Geometry check sheet. Reference: the model listing, model coordinates, mm. A direction names the side the tool comes from. Round coordinates to 2 decimals unless told otherwise and drop trailing zeros. Order: outer loops, then holes, each group sorted by start corner. A loop starts at its lowest first (then second) coordinate and runs counter-clockwise, first axis right, second up. Notation, with made-up numbers: (65, 79.25) - (105, 79.25) arc R10 ccw to (105, 86.25) - close; hole circle Ø2 at (-32.5, 67). An arc over 180 degrees is marked (long way). Return JSON: item names as keys, results as strings. Group by question number.
Q1. Draft check along Y on faces 6 (the flat face through (113.5, 13, 5)), 7 (the flat face through (-2, 2, -10)), 8 (the flat face through (-2, 0, 0)), 9 (the flat face through (-2, 26, 5)). Enter one of: pulls with the +Y half, pulls with the -Y half, needs draft (parallel to the pull), parting line crosses it, or undercut.
Q2. Sectioned sample at B-B, the plane x = 70. Record the cut outline in (y, z), then the cut area to 3 significant figures.
Q3. Sectioned sample at A-A, the plane y = 15.75. Record the cut outline in (x, z), then the cut area to 3 significant figures.
Q4. Material ranges on line 1 along X through (y, z) = (9.25, 1); line 2 along Z through (x, y) = (-26.9, 2.35); line 3 along Y through (x, z) = (-119.5, 3.5), recorded low to high.
Q5. Gauge pin test, flat ends, axial feed: pin 1 Ø6.5 at (x, y) = (-58.5, 20.5) entering from -Z; pin 2 Ø1 at (x, z) = (-17, -1.5) entering from +Y. Record the tip position at first contact, or that the pin passes through.
Q6. Tool access check on faces 1 (the flat face through (-2, 16, 0)), 2 (the flat face through (-2, 5, -4)), 3 (the flat face through (-2, 13, 10)), 4 (the flat face through (134.5, 13, 5)), 5 (the flat face through (121, 21, 5)). Record the directions out of +Z, -Z, +X, -X, +Y, -Y that give a thin tool (end or side, any length) a straight path to the whole face; none if there is none.
```python
from build123d import *

# Parameters (mm, degrees)
SKETCH_W     = 269
SKETCH_H     = 26
SKETCH_W_2   = 16
SKETCH_H_2   = 16
PAD_DEPTH    = 10
SKETCH002_W  = 269
SKETCH002_H  = 5
PAD001_DEPTH = 10
SKETCH003_R  = 1.5
POCKET_DEPTH = 5.001


with BuildPart() as part:
    # Sketch → Pad (new body)
    with BuildSketch(Plane.XY):
        with Locations((0, 13)):
            Rectangle(SKETCH_W, SKETCH_H)
        with Locations((121.5, 13)):
            Rectangle(SKETCH_W_2, SKETCH_H_2, mode=Mode.SUBTRACT)
        with Locations((-121.5, 13)):
            Rectangle(SKETCH_W_2, SKETCH_H_2, mode=Mode.SUBTRACT)
    extrude(amount=PAD_DEPTH)

    # Sketch002 (on Face13 of Pad) → Pad001 (join)
    with BuildSketch(Plane(origin=(0, 0, 0), x_dir=(1, 0, 0), z_dir=(0, 0, -1))):
        with Locations((0, -2.5)):
            Rectangle(SKETCH002_W, SKETCH002_H)
    extrude(amount=PAD001_DEPTH)

    # Sketch003 (on Face9 of Pad001) → Pocket (cut, through all)
    with BuildSketch(Plane(origin=(0, 5, 0), x_dir=(-1, 0, 0), z_dir=(0, 1, 0))):
        with Locations((-134.5, -5)):
            Circle(SKETCH003_R)
        with Locations((-80.7, -5)):
            Circle(SKETCH003_R)
        with Locations((-26.9, -5)):
            Circle(SKETCH003_R)
        with Locations((26.9, -5)):
            Circle(SKETCH003_R)
        with Locations((80.7, -5)):
            Circle(SKETCH003_R)
        with Locations((134.5, -5)):
            Circle(SKETCH003_R)
    extrude(amount=-POCKET_DEPTH, mode=Mode.SUBTRACT)


solid = part.part
```
Reply:
{
 "1": {"face 6": "undercut", "face 7": "needs draft", "face 8": "pulls with the -Y half", "face 9": "pulls with the +Y half"},
 "2": {"outline": "(0, -10) - (5, -10) - (5, 0) - (26, 0) - (26, 10) - (0, 10) - close", "area": "310 mm^2"},
 "3": {"outline": "(-134.5, 0) - (-129.5, 0) - (-129.5, 10) - (-134.5, 10) - close; (-113.5, 0) - (113.5, 0) - (113.5, 10) - (-113.5, 10) - close; (129.5, 0) - (134.5, 0) - (134.5, 10) - (129.5, 10) - close", "area": "2,370 mm^2"},
 "4": {"line 1": "-134.5 to -129.5, -113.5 to 113.5, 129.5 to 134.5", "line 2": "-10 to -6.5, -3.5 to 10", "line 3": "0 to 5, 21 to 26"},
 "5": {"pin 1": "z = 0", "pin 2": "y = 5"},
 "6": {"face 1": "-Z, +X, -X, +Y", "face 2": "-Z", "face 3": "+Z, +X, -X, +Y, -Y", "face 4": "+Z, -Z, +X, +Y, -Y", "face 5": "+Z, -Z"}
}
